```python
from build123d import *

# Parameters (mm, degrees)
SKETCH1_R           = 2.6375
BOSS_EXTRUDE1_DEPTH = 4


with BuildPart() as part:
    # Sketch1 → Boss-Extrude1 (new body)
    with BuildSketch(Plane.XZ):
        with BuildLine():
            Line((91.828846411, -34.604196587), (83.987808778, -41.556583288))
            ThreePointArc((83.987808778, -41.556583288), (83.299503374, -41.95543418), (82.510169812, -42.054423534))
            ThreePointArc((82.510169812, -42.054423534), (78.551510946, -51.744694217), (87.430169632, -46.200170264))
            ThreePointArc((87.430169632, -46.200170264), (87.461256355, -45.116261185), (88.053439291, -44.207886459))
            Line((88.053439291, -44.207886459), (93.937481824, -39.062233577))
            ThreePointArc((93.937481824, -39.062233577), (94.910198817, -38.597536781), (95.982821704, -38.705247518))
            ThreePointArc((95.982821704, -38.705247518), (102.625664422, -30.628415987), (92.497951624, -33.234562654))
            ThreePointArc((92.497951624, -33.234562654), (92.299001629, -33.985625361), (91.828846411, -34.604196587))
        make_face()
        with Locations((82.095552315, -47.538773298)):
            Circle(SKETCH1_R, mode=Mode.SUBTRACT)
        with Locations((97.986880619, -33.583358427)):
            Circle(SKETCH1_R, mode=Mode.SUBTRACT)
    extrude(amount=-BOSS_EXTRUDE1_DEPTH)


solid = part.part
```
Build history of the part. All positions in model axes, mm. Round coordinates to 2 decimals unless told otherwise and drop trailing zeros. Write each loop counter-clockwise with the first axis right and the second up, starting at its lowest first coordinate (ties: lowest second). Pieces come first, ordered by that corner, then holes.
1) Band-saw the part on D-D, the plane z = -43.75. List the corners of the cut face in (x, y).
2) Drill centre lines: probe 1 along Z at (x, y) = (81, 0.4); probe 2 along Z at (x, y) = (84, 0.3); probe 3 along X at (y, z) = (3.05, -31.5). Where is each one in solid material? Low to high.
3) Pin check, flat tips, straight feed: pin 1 (2 mm diameter, centred on y = 2, z = -45.5, fed in from +X); pin 2 (4.5 mm diameter, centred on x = 82.1, z = -47.54, fed in from -Y). Stop position of each tip, or through.
4) Mould opens along X. For faces 1 (the cylindrical face through (92.3, 1.97, -33.98)), 2 (the cylindrical face through (87.457, 1.972, -45.131)), 3 (the flat face through (89, 0, -41)), 4 (the cylindrical face through (83.513, 1.972, -45.315)) say: +X half, -X half, draft (parallel to the pull), parting line (faces both ways), or undercut.
5) Band-saw the part on A-A, the plane z = -49. List the corners of the cut face in (x, y), and give its area (3 significant figures).
6) Band-saw the part on C-C, the plane y = 0.65. List the corners of the cut face in (x, z) (1 decimal).
7) Band-saw the part on B-B, the plane x = 80.25. List the corners of the cut face in (y, z).
Ans:
1. outline: (78.11, 0) - (88.58, 0) - (88.58, 4) - (78.11, 4) - close
2. probe 1: z = -52.93 to -49.94, -45.14 to -42.15
2. probe 2: z = -52.7 to -49.36, -45.71 to -41.55
2. probe 3: x = 92.9 to 96.37, 99.6 to 103.08
3. pin 1: stops at x = 87.78
3. pin 2: passes through
4. face 1: -X half
4. face 2: +X half
4. face 3: draft
4. face 4: undercut
5. outline: (76.79, 0) - (79.9, 0) - (79.9, 4) - (76.79, 4) - close; (84.29, 0) - (87.4, 0) - (87.4, 4) - (84.29, 4) - close
5. area: 24.9 mm2
6. outline: (82.5, -42.1) arc R5.5 ccw (long way) to (87.4, -46.2) arc R2 cw to (88.1, -44.2) - (93.9, -39.1) arc R2 cw to (96, -38.7) arc R5.5 ccw (long way) to (92.5, -33.2) arc R2 cw to (91.8, -34.6) - (84, -41.6) arc R2 cw to start; hole circle Ø5.3 at (82.1, -47.5); hole circle Ø5.3 at (98, -33.6)
7. outline: (0, -52.72) - (4, -52.72) - (4, -49.42) - (0, -49.42) - close; (0, -45.65) - (4, -45.65) - (4, -42.36) - (0, -42.36) - close
